Verification items for the finished model (mm, model axes). A direction names the side the tool comes from. Coordinates: 2 decimals unless noted, no trailing zeros. Order: outer loops, then holes, each group sorted by start corner. A loop starts at its lowest first (then second) coordinate and runs counter-clockwise, first axis right, second up. Notation, with made-up numbers: M -28.75,27 L 23.25,27 A8 ccw 23.25,32 Z; hole C 3.25,83.5 d1. An arc over 180 degrees is marked long. Return JSON: item names as keys, results as strings.
```python
from build123d import *

# Parameters (mm, degrees)
F2_W        = 38.7379527092
F2_H        = 101.6
F2_H_2      = 2.0811606664
F3_DEPTH    = 65.278
F4_T2_ANGLE = 342.3977360444
F4_T4_ANGLE = 26.640456748


# Not quite as in the source:
# - a fillet or chamfer that OpenCascade refuses, or shapes differently, is made with other operations: its cross-section is extruded or revolved along the edge and cut away or added
# - a feature names something its author has since deleted; it is built from what else it names


with BuildPart() as f1:
    # F0 (on Front) → F1 (revolve)
    with BuildSketch(Plane.XZ):
        Polygon((-19.05, -101.1886583478), (-19.05, -113.8886583478), (69.85, -113.8886583478), (69.85, -101.1886583478), (9.1183487131, -101.1886583478), (5.3083487131, -101.1886583478), align=None)
        Polygon((5.3083487131, 21.6246411156), (5.3083487131, -101.1886583478), (9.1183487131, -101.1886583478), (9.1183487131, 25.8113416522), align=None)
        Polygon((0, 15.7914478332), (5.3083487131, 21.6246411156), (9.1183487131, 25.8113416522), (68.3819557915, 90.9344323502), (68.3744283423, 94.5670089535), (-0.0075274492, 19.4240244364), (-11.8764168927, 6.3816397113), (-12.0276177274, 2.5746411156), align=None)
    revolve(axis=Axis((-19.05, 0, -107.5386583478), (0, 0, 1)))

    # F2 (on Right) → F3 (cut, symmetric)
    with BuildSketch(Plane.YZ):
        with Locations((-19.3689763546, -50.8)):
            Rectangle(F2_W, F2_H)
        with Locations((-19.3689763546, 1.0405803332)):
            Rectangle(F2_W, F2_H_2)
    extrude(amount=F3_DEPTH, both=True, mode=Mode.SUBTRACT)

    # F4: fillet of radius 5.08 on 1 edges, made by hand

    # F4_s1 → F4_t2 (revolve, cut)
    with BuildSketch(Plane.XZ):
        with BuildLine():
            ThreePointArc((69.85, -106.2686583478), (68.3621024484, -102.6765558993), (64.77, -101.1886583478))
            Line((64.77, -101.1886583478), (69.85, -101.1886583478))
            Line((69.85, -101.1886583478), (69.85, -106.2686583478))
        make_face()
    revolve(axis=Axis((-19.05, 0, -101.1886583478), (0, 0, 1)), revolution_arc=F4_T2_ANGLE, mode=Mode.SUBTRACT)

    # F4_s3 → F4_t4 (revolve, cut)
    with BuildSketch(Plane(origin=(-3.8300767646, -7.635016329, 0), x_dir=(0, 0, 1), z_dir=(-0.4483903416, -0.8938378497, 0))):
        with BuildLine():
            ThreePointArc((-106.2686583478, -71.8723889628), (-102.6765558993, -70.3844914112), (-101.1886583478, -66.7923889628))
            Line((-101.1886583478, -66.7923889628), (-101.1886583478, -71.8723889628))
            Line((-101.1886583478, -71.8723889628), (-106.2686583478, -71.8723889628))
        make_face()
    revolve(axis=Axis((-19.05, 0, -101.1886583478), (0, 0, 1)), revolution_arc=F4_T4_ANGLE, mode=Mode.SUBTRACT)


solid = f1.part
```
Q1. Tool access check on faces 4 (the face through (-22.22, 24.15, -40.64)), 5 (the face through (-38, -85.35, 92.78)), 6 (the face through (-19, 10, -101.189)), 7 (the face through (-18, 1, -113.889)). Record the directions out of +Z, -Z, +X, -X, +Y, -Y that give a thin tool (end or side, any length) a straight path to the whole face; none if there is none.
Values:
{"face 4": "none", "face 5": "+Z", "face 6": "-Y", "face 7": "-Z, +X, -X, +Y, -Y"}
Q2. Cross-section at B-B, the plane z = 54.5. Record the boundary of the cut face in (x, y), and give its area (3 significant figures).
Values:
{"outline": "C -19.05,0 d108.55; hole C -19.05,0 d101.92", "area": "1,100 mm^2"}
Q3. Draft check along Y on faces 1 (the face through (-19, -25, 2.081)), 2 (the face through (-24.669, -4.308, 4.028)), 3 (the face through (65.745, 26.703, -110.025)). Enter one of: pulls with the +Y half, pulls with the -Y half, needs draft (parallel to the pull), parting line crosses it, or undercut.
Values:
{"face 1": "needs draft", "face 2": "undercut", "face 3": "parting line crosses it"}
Q4. Material ranges on line 1 along Y through (x, z) = (-19.05, -32); line 2 along Z through (x, y) = (-46, -49.5); line 3 along Z through (x, y) = (-58.5, -43), recorded low to high.
Values:
{"line 1": "24.36 to 28.17", "line 2": "-113.89 to -101.19, 56.79 to 60.43", "line 3": "-113.89 to -101.19, 58.98 to 62.62"}
Q5. Cross-section at A-A, the plane z = -48. Record the boundary of the cut face in (x, y).
Values:
{"outline": "M -47.22,0 L -43.41,0 A24.36 cw 5.31,0 L 9.12,0 A28.17 ccw Z"}
Q6. Go/stop test with flat-tipped pins: pin 1 (1.5 mm diameter, centred on x = 17, y = -38, fed in from +Z); pin 2 (12 mm diameter, centred on x = 25, y = 56, fed in from +Z); pin 3 (7.5 mm diameter, centred on x = -27.5, y = 8, fed in from +Z). Record where each tip stops, or that it passes through.
Values:
{"pin 1": "z = 56.88", "pin 2": "z = 83.39", "pin 3": "z = 15.41"}
